Here's the drawing with two shaded views (mm, measured from the low corner). I have some questions. Give positions to 0.01 mm unless a question says otherwise; leave off trailing zeros. Loops run counter-clockwise (first coordinate to the right, second up) from the corner with the lowest first, then second, coordinate; pieces in that order, holes last.
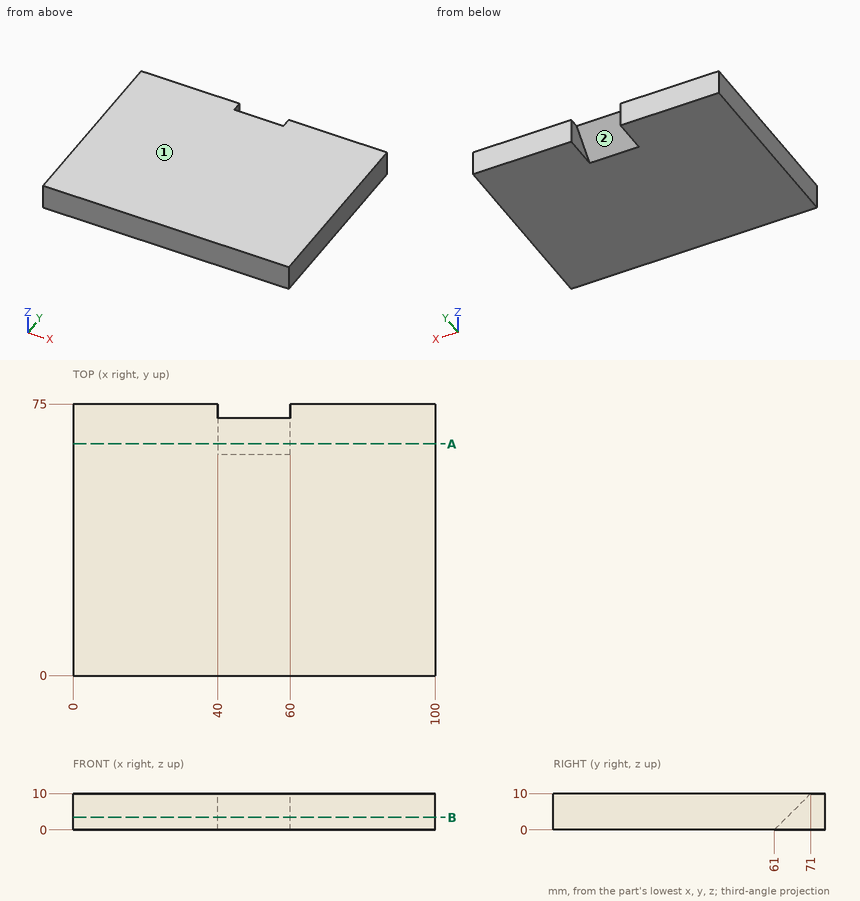
(1) Suppose I cut it at A-A on y = 64. List the corners of the cut face in (x, z) for me.
Returned:
outline: (0, 0) - (40, 0) - (40, 3) - (60, 3) - (60, 0) - (100, 0) - (100, 10) - (0, 10) - close
(2) Please list where these lines run through material, in increasing order: probe 1 along X at (y, z) = (70.5, 9); probe 2 along Y at (x, z) = (49, 4.5); probe 3 along Y at (x, z) = (41, 5.25).
Returned:
probe 1: x = 0 to 40, 60 to 100
probe 2: y = 0 to 65.5
probe 3: y = 0 to 66.25
(3) Thinking about a two-plate mould opening in X: for the marked faces 1 and 2, which applies, pulls with the +X half, pulls with the -X half, needs draft (parallel to the pull), parting line crosses it, or undercut?
Returned:
face 1: needs draft
face 2: undercut
(4) Suppose I cut it at B-B on z = 3.5. List the corners of the cut face in (x, y) for me, plus the area to 3 significant figures.
Returned:
outline: (0, 0) - (100, 0) - (100, 75) - (60, 75) - (60, 64.5) - (40, 64.5) - (40, 75) - (0, 75) - close
area: 7,290 mm2
